The model under review builds one solid part; all positions refer to its coordinate system, in mm. A direction names the side the tool comes from. Coordinates: 2 decimals unless noted, no trailing zeros. Order: outer loops, then holes, each group sorted by start corner. A loop starts at its lowest first (then second) coordinate and runs counter-clockwise, first axis right, second up. Notation, with made-up numbers: (10, 59) -> (37, 59) arc R28 ccw to (37, 97) -> close; hole circle Ø6 at (33.5, 21.25). An arc over 180 degrees is marked (long way). Use one line per item in the form item = value.
from build123d import *

# Parameters (mm, degrees)
PAD_DEPTH    = 20
PAD001_DEPTH = 30


with BuildPart() as pad:
    # Sketch → Pad (new body)
    with BuildSketch(Plane.XY):
        Polygon((-35, -30), (35, -30), (35, -95), (14.792741, -130), (10, -130), (10, -60), (-10, -60), (-10, -130), (-14.792741, -130), (-35, -95), align=None)
    extrude(amount=PAD_DEPTH)


with BuildPart() as fusion:
    # Sketch001 → Pad001 (new body)
    with BuildSketch(Plane.XZ):
        Polygon((-35, 0), (35, 0), (35, 50), (10, 50), (18.660254, 35), (-18.660254, 35), (-10, 50), (-35, 50), align=None)
    extrude(amount=PAD001_DEPTH)

    # Fusion: union Pad
    add(pad.part)


solid = fusion.part
Item 1: We need section D-D (x = 11.5). Write out the cut boundary in (y, z).
Results found:
outline = (-130, 0) -> (0, 0) -> (0, 35) -> (-30, 35) -> (-30, 20) -> (-130, 20) -> close; (-30, 47.4) -> (0, 47.4) -> (0, 50) -> (-30, 50) -> close
Item 2: To check wall thickness, follow L1, parallel to Y at x = -25, z = 38; L2, parallel to Y at x = -4, z = 7; L3, parallel to Z at x = -15, y = -94.5. State the ranges of each line that lie inside material, in increasing order. Write a range as from..to.
Results found:
L1 = -30..0
L2 = -60..0
L3 = 0..20
Item 3: We need section C-C (y = -10.5). Write out the cut boundary in (x, z), plus the area to 3 significant figures.
Results found:
outline = (-35, 0) -> (35, 0) -> (35, 50) -> (10, 50) -> (18.66, 35) -> (-18.66, 35) -> (-10, 50) -> (-35, 50) -> close
area = 3,070 mm²
Item 4: We need section B-B (z = 47). Write out the cut boundary in (x, y).
Results found:
outline = (-35, -30) -> (-11.73, -30) -> (-11.73, 0) -> (-35, 0) -> close; (11.73, -30) -> (35, -30) -> (35, 0) -> (11.73, 0) -> close
Item 5: Clearance check with flat-ended pins moving along their axes: pin 1 (3 mm diameter, centred on x = 23.5, y = -59, fed in from -Z); pin 2 (8 mm diameter, centred on x = 14, y = -104.5, fed in from +Z); pin 3 (22 mm diameter, centred on y = -112.5, z = 14.5, fed in from -X); pin 4 (15 mm diameter, centred on x = 8.5, z = 31, fed in from -Y). State where each tip first meets the part, or that it passes through.
Results found:
pin_1 = 0
pin_2 = 20
pin_3 = -31.25
pin_4 = -30
Item 6: Draft analysis for pull direction Z (two halves, no side actions). For faces 6 (the face through (0, -50, 0)), 7 (the face through (0, -15, 35)), 8 (the face through (25.038, -112.255, 9.86)), state which applies: released by +Z, released by -Z, zero draft, split by the parting line, or undercut.
Results found:
face_6 = released by -Z
face_7 = undercut
face_8 = zero draft
Item 7: Tool access review of faces 1 (the face through (-14.39, -14.79, 42.4)), 2 (the face through (-12, -130, 10)), 3 (the face through (23, -15, 50)), 4 (the face through (10, -95, 10)), 5 (the face through (0, -30, 32)): name each direction out of +Z, -Z, +X, -X, +Y, -Y from which nothing blocks a thin tool from reaching the whole face with its end or side.
Results found:
face_1 = +Y, -Y
face_2 = +Z, -Z, +X, -X, -Y
face_3 = +Z, +X, -X, +Y, -Y
face_4 = +Z, -Z, -Y
face_5 = +Z, +X, -X, -Y
Item 8: We need section A-A (y = -69). Write out the cut boundary in (x, z), plus the area to 3 significant figures.
Results found:
outline = (-35, 0) -> (-10, 0) -> (-10, 20) -> (-35, 20) -> close; (10, 0) -> (35, 0) -> (35, 20) -> (10, 20) -> close
area = 1,000 mm²
